The listing builds one solid part. Answer for the finished solid, in the listing's coordinates (mm). A direction names the side the tool comes from. Coordinates: 2 decimals unless noted, no trailing zeros. Write each loop counter-clockwise with the first axis right and the second up, starting at its lowest first coordinate (ties: lowest second). Pieces come first, ordered by that corner, then holes.
(1) Given P1, Ø4, axis at x = 40, z = 4.5, coming from the -Y side, flat-ended and moving along its own axis, determine where the tip first touches the part or whether it passes through.
(2) The part is cut by section B-B on z = 17. Determine the outline of the cut face in (x, y).
(3) The part is cut by section C-C on x = 87. Determine the outline of the cut face in (y, z).
(4) Which of the six approach directions +Z, -Z, +X, -X, +Y, -Y give full straight-line access (tool end or side, diameter ignored) to faces 1 (the flat face through (68, 67, 0)), 2 (the flat face through (19.05, 31, 10))?
(5) For a pull along Y with two mould halves and no side action, classify faces 3 (the flat face through (9, 0, 9)), 4 (the flat face through (68, 81.05, 9)), 5 (the flat face through (138.1, 40, 10)) as +Y half, -Y half, draft (parallel to the pull), parting line (faces both ways), or undercut.
(6) The part is cut by section A-A on y = 21.5. Determine the outline of the cut face in (x, z).
(7) Straight lines are drawn through the part: line 1 (X direction, y = 16, z = 16.5); line 2 (Y direction, x = 84.5, z = 8). For each, find the intervals that lie inside material, in ascending order.
from build123d import *

# Parameters (mm, degrees)
SKETCH2_W             = 19.05
SKETCH2_H             = 19.05
BOSS_EXTRUDE1_DEPTH   = 62
BOSS_EXTRUDE1_2_DEPTH = 62
SKETCH3_W             = 138.1
SKETCH3_H             = 19.05
BOSS_EXTRUDE2_DEPTH   = 19.05


with BuildPart() as part:
    # Sketch2 → Boss-Extrude1 (new body)
    with BuildSketch(Plane(origin=(0, 0, 0), x_dir=(1, 0, 0), z_dir=(0, 1, 0))):
        with Locations((9.525, -9.525)):
            Rectangle(SKETCH2_W, SKETCH2_H)
    extrude(amount=BOSS_EXTRUDE1_DEPTH)



with BuildPart() as body_2:
    # Sketch2 → Boss-Extrude1 2 (new body)
    with BuildSketch(Plane(origin=(0, 0, 0), x_dir=(1, 0, 0), z_dir=(0, 1, 0))):
        with Locations((128.575, -9.525)):
            Rectangle(SKETCH2_W, SKETCH2_H)
    extrude(amount=BOSS_EXTRUDE1_2_DEPTH)


with BuildPart() as part_1:
    add(part.part)

    add(body_2.part)  # Boss-Extrude2 merges body 2
    # Sketch3 → Boss-Extrude2 (add)
    with BuildSketch(Plane(origin=(0, 62, 0), x_dir=(1, 0, 0), z_dir=(0, 1, 0))):
        with Locations((69.05, -9.525)):
            Rectangle(SKETCH3_W, SKETCH3_H)
    extrude(amount=BOSS_EXTRUDE2_DEPTH)


solid = part_1.part
Model answer:
1. P1: stops at y = 62
2. outline: (0, 0) - (19.05, 0) - (19.05, 62) - (119.05, 62) - (119.05, 0) - (138.1, 0) - (138.1, 81.05) - (0, 81.05) - close
3. outline: (62, 0) - (81.05, 0) - (81.05, 19.05) - (62, 19.05) - close
4. face 1: -Z, +X, -X, +Y, -Y
4. face 2: +Z, -Z, -Y
5. face 3: -Y half
5. face 4: +Y half
5. face 5: draft
6. outline: (0, 0) - (19.05, 0) - (19.05, 19.05) - (0, 19.05) - close; (119.05, 0) - (138.1, 0) - (138.1, 19.05) - (119.05, 19.05) - close
7. line 1: x = 0 to 19.05, 119.05 to 138.1
7. line 2: y = 62 to 81.05
